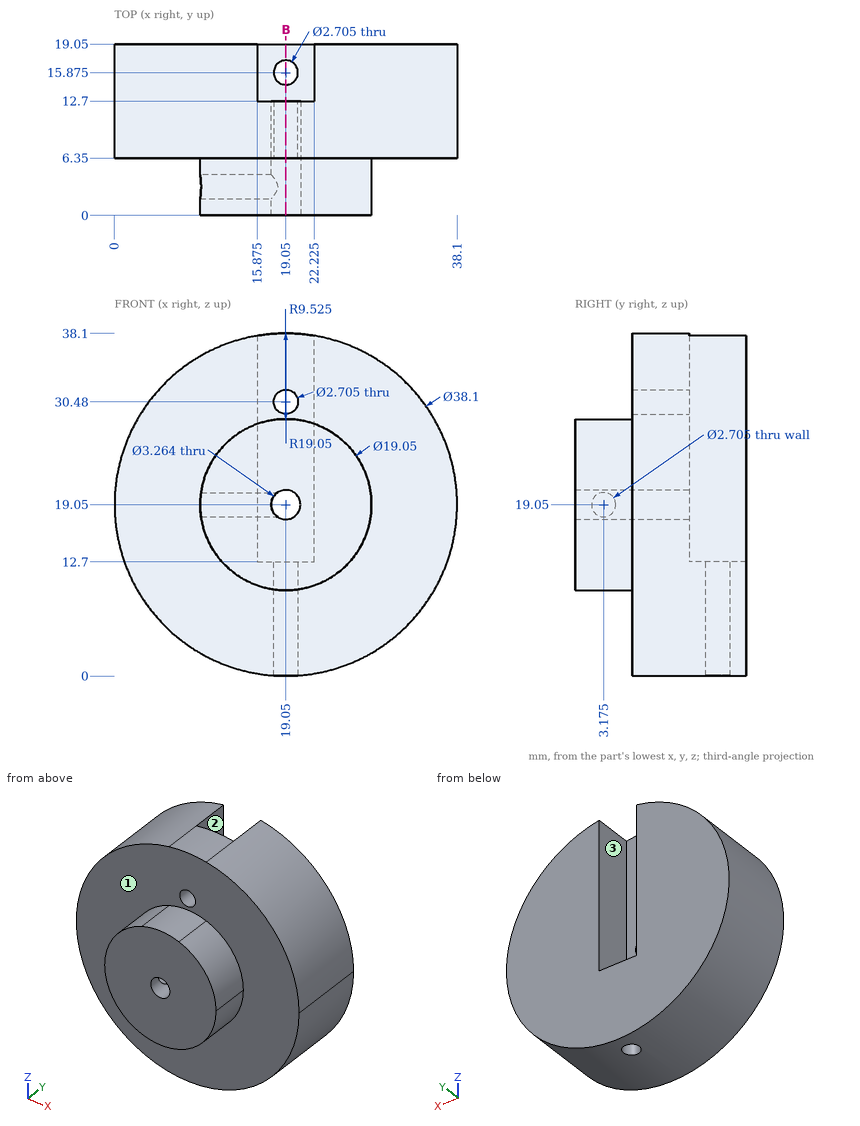
The figure shows three views and two pictorial views of one solid part (mm, origin at its lowest corner). Answer the questions. Round coordinates to 2 decimals unless told otherwise and drop trailing zeros. Write each question's results on one line, items separated by ' | '.
Q1. Straight lines are drawn through the part: line 1 along Y through (x, z) = (19.05, 6.25); line 2 along Y through (x, z) = (14, 19); line 3 along Y through (x, z) = (15, 9.5). For each, find the intervals that lie inside material, in ascending order. Write a range as [from, to].
Data:
line 1: [6.35, 14.52], [17.23, 19.05] | line 2: [0, 1.82], [4.53, 19.05] | line 3: [6.35, 19.05]
Q2. Flat-ended cylindrical pins translate along their axes: P1, Ø10, axis at y = 8.5, z = 15, coming from the -X side; P2, Ø1.9, axis at y = 16.5, z = 27.5, coming from the -X side; P3, Ø1.6, axis at y = 3.175, z = 19.05, coming from the +X side (3 decimals); P4, Ø1.9, axis at y = 17, z = 29, coming from the +X side. Find the tip coordinate at first contact, or state that the pin passes through.
Data:
P1: x = 0 | P2: x = 1.54 | P3: x = 28.575 | P4: x = 35.84
Q3. Determine the mould class of the marked faces 1, 2 and 3 for opening direction X: released by +X, released by -X, zero draft, split by the parting line, or undercut.
Data:
face 1: zero draft | face 2: undercut | face 3: undercut
Q4. Section B-B, the plane x = 19.05 is taken. Give the number of separate pieces and of enclosed holes in the cut face, then the cut area to 3 significant figures.
Data:
separate pieces: 4 | enclosed holes: 0 | area: 351 mm^2
